from build123d import *

# Parameters (mm, degrees)
F0_R     = 3.1875
F1_DEPTH = 0.7
F2_R     = 0.6
F3_DEPTH = 25
F4_R     = 0.34999
F5_R     = 0.25
F6_DEPTH = 1


# Not quite as in the source:
# - a fillet or chamfer is up to 0.001 mm smaller than in the source, because OpenCascade refuses the exact size


with BuildPart() as f1:
    # F0 (on Front) → F1 (new body)
    with BuildSketch(Plane.XZ):
        Circle(F0_R)
    extrude(amount=F1_DEPTH)

    # F2 (on face) → F3 (cut)
    with BuildSketch(Plane.XZ.offset(0.7)):
        Circle(F2_R)
    extrude(amount=-F3_DEPTH, mode=Mode.SUBTRACT)

    # F4 (radius 0.35 in the source; OpenCascade refuses exactly that, so slightly less here)
    f4_edges = [f1.edges().sort_by_distance(p)[0] for p in [
        (3.1875, -0.35, 0),
        (-3.1875, 0, 0),
        (-3.1875, -0.7, 0),
    ]]
    fillet(f4_edges, radius=F4_R)

    # F5 (on face) → F6 (join)
    with BuildSketch(Plane.XZ.offset(0.7)):
        with Locations((0, 2.2993473568)):
            Circle(F5_R)
    extrude(amount=F6_DEPTH)


solid = f1.part
Verification items for the finished model (mm, model axes). Round coordinates to 2 decimals unless told otherwise and drop trailing zeros. Loops run counter-clockwise (first coordinate to the right, second up) from the corner with the lowest first, then second, coordinate; pieces in that order, holes last. Notation, with made-up numbers: (46, 23.5) - (92, 23.5) arc R22 ccw to (92, 51.5) - close; hole circle Ø5 at (88, 62). An arc over 180 degrees is marked (long way). Answer in a Markdown table with one row per item. Add a question column.
Q1. Section check C-C on y = -0.5. Enter the section's corners in (x, z), plus the area to 3 significant figures.
Q2. Gauge pin test, flat end, axial feed: pin 1 (1.7 mm diameter, centred on x = 1.5, z = -0.5, fed in from -Y). Record the tip position at first contact, or that the pin passes through.
Q3. Material ranges on line 1 (Y direction, x = -1.5, z = 2.25); line 2 (Z direction, x = 0, y = -0.15); line 3 (Z direction, x = 0, y = -1.35), recorded low to high.
Q4. Release check for a two-part mould opening along X. For faces 1 (the face through (0.323, -0.355, 0.506)), 2 (the face through (0, 0, 1)) record: pulls with the +X half, pulls with the -X half, needs draft (parallel to the pull), parting line crosses it, or undercut.
Found:
| question | item | result |
|---|---|---|
| 1 | outline | circle Ø6.31 at (0, 0); hole circle Ø1.2 at (0, 0) |
| 1 | area | 30.1 mm² |
| 2 | pin 1 | stops at y = -0.7 |
| 3 | line 1 | y = -0.7 to 0 |
| 3 | line 2 | z = -3.12 to -0.6, 0.6 to 3.12 |
| 3 | line 3 | z = 2.05 to 2.55 |
| 4 | face 1 | undercut |
| 4 | face 2 | needs draft |
